Input: part model. Units: mm. Frame: model coordinates. A direction names the side the tool comes from. Round coordinates to 2 decimals unless told otherwise and drop trailing zeros. Loops run counter-clockwise (first coordinate to the right, second up) from the corner with the lowest first, then second, coordinate; pieces in that order, holes last. Notation, with made-up numbers: (34, 39) -> (49, 39) arc R16 cw to (49, 63) -> close; hole circle Ø11 at (16.5, 70.5). An arc over 180 degrees is marked (long way). Answer as a JSON object with one key per item and string values. Group by question number.
Item 1: Section query C-C on z = 15.25. Count the separate pieces of the cut face and the enclosed holes in it, and give its area (3 significant figures).
Item 2: Material intervals for line 1 (Y direction, x = 44, z = 6.75); line 2 (X direction, y = 22, z = 8.5); line 3 (X direction, y = 12, z = 15), sorted ascending. Write a range as [from, to].
Item 3: Section query B-B on y = 7.5. Return loops of the section in (x, z), and give its area (3 significant figures).
Item 4: Pin query (flat end, axial travel): pin 1 (19 mm diameter, centred on x = 2, y = 84, fed in from -Z); pin 2 (1.5 mm diameter, centred on x = 32, y = 17.5, fed in from -Z); pin 3 (1 mm diameter, centred on y = -23.5, z = 7, fed in from -X); pin 4 (2 mm diameter, centred on x = -16, z = 21.5, fed in from +Y). Return the tip coordinate at first contact, or that it passes through.
Item 5: Section query A-A on x = 18. Return loops of the section in (y, z), and give its area (3 significant figures).
Item 6: Set-up query: faces 3 (the cylindrical face through (-0.16, 87.21, 22.48)), 4 (the flat face through (-2, 85, 12)), 5 (the cylindrical face through (-0.19, 87.21, 3.04)), 6 (the flat face through (-1, -31.105, 12)). Return all of +Z, -Z, +X, -X, +Y, -Y with unobstructed straight access to the full face (end or side cutting, diameter ignored); none if empty.
Item 7: Draft query along Y for faces 1 (the flat face through (-20.54, 66.63, 18.6)), 2 (the flat face through (-30, 13, 0)). Return one class per face: released by +Y, released by -Y, zero draft, split by the parting line, or undercut.
from build123d import *

# Parameters (mm, degrees)
PAD_DEPTH             = 24
POCKET_DEPTH          = 3
SKETCH002_W           = 70
SKETCH002_H           = 18.5
POCKET001_DEPTH       = 18
POLARPATTERN_COUNT    = 3
POCKET002_DEPTH       = 6
CHAMFER_SIZE          = 8
FILLET_R              = 13
FILLET001_R           = 11
CHAMFER001_SIZE       = 16.1
FILLET002_R           = 11
FILLET003_R           = 12
POCKET003_DEPTH       = 6
POCKET004_DEPTH       = 18
POCKET005_DEPTH       = 21.001
SKETCH007_W           = 15.5
SKETCH007_H           = 15
POCKET006_DEPTH       = 5
SKETCH010_W           = 13.6
SKETCH010_H           = 9
POCKET009_DEPTH       = 15.5
POCKET010_DEPTH       = 3
SKETCH012_R           = 1.85
SKETCH012_R_2         = 0.99
POCKET011_DEPTH       = 498.0492855781
POLARPATTERN001_COUNT = 3


with BuildPart() as part:
    # Sketch → Pad (new body)
    with BuildSketch(Plane.XY):
        Polygon((0, 112.2094915052), (-97.1762701892, -56.1047457526), (97.1762701892, -56.1047457526), align=None)
        Polygon((0, 62.2094915052), (-53.875, -31.1047457526), (53.875, -31.1047457526), align=None, mode=Mode.SUBTRACT)
    extrude(amount=PAD_DEPTH)

    # Sketch001 (on Face8 of Pad) → Pocket (cut)
    with BuildSketch(Plane.XY.offset(24)):
        Polygon((0, 98.2094915052), (-85.0519145362, -49.1047457526), (85.0519145362, -49.1047457526), align=None)
        Polygon((0, 76.2094915052), (-65.999355653, -38.1047457526), (65.999355653, -38.1047457526), align=None, mode=Mode.SUBTRACT)
    extrude(amount=-POCKET_DEPTH, mode=Mode.SUBTRACT)

    # Sketch002 (on Face4 of Pocket) → Pocket001 (cut)
    with BuildSketch(Plane(origin=(0, 0, 0), x_dir=(1, 0, 0), z_dir=(0, 0, -1))):
        with Locations((0, 43.6047457526)):
            Rectangle(SKETCH002_W, SKETCH002_H)
    pocket001 = extrude(amount=-POCKET001_DEPTH, mode=Mode.SUBTRACT)

    # PolarPattern: Pocket001 ×3 about axis
    polarpattern_axis = Axis((0, 0, 0), (0, 0, -1))
    for i in range(1, POLARPATTERN_COUNT):
        add(pocket001.rotate(polarpattern_axis, i * 360 / POLARPATTERN_COUNT), mode=Mode.SUBTRACT)

    # Sketch003 (on Face4 of PolarPattern) → Pocket002 (cut)
    with BuildSketch(Plane(origin=(0, 0, 0), x_dir=(1, 0, 0), z_dir=(0, 0, -1))):
        Polygon((0, -100.2094915052), (86.7839653438, 50.1047457526), (-86.7839653438, 50.1047457526), align=None)
        Polygon((0, -74.2094915052), (64.2673048454, 37.1047457526), (-64.2673048454, 37.1047457526), align=None, mode=Mode.SUBTRACT)
    extrude(amount=-POCKET002_DEPTH, mode=Mode.SUBTRACT)

    # Chamfer
    chamfer_edges = [part.edges().sort_by_distance(p)[0] for p in [
        (-53.875, -31.104746, 12),
        (53.875, -31.104746, 12),
        (0, 62.209492, 12),
    ]]
    chamfer(chamfer_edges, length=CHAMFER_SIZE)

    # Fillet
    fillet_edges = [part.edges().sort_by_distance(p)[0] for p in [
        (0, 100.209492, 3),
        (-86.783965, -50.104746, 3),
        (86.783965, -50.104746, 3),
    ]]
    fillet(fillet_edges, radius=FILLET_R)

    # Fillet001
    fillet001_edges = [part.edges().sort_by_distance(p)[0] for p in [
        (0, 74.209492, 3),
        (64.267305, -37.104746, 3),
        (-64.267305, -37.104746, 3),
    ]]
    fillet(fillet001_edges, radius=FILLET001_R)

    # Chamfer001
    chamfer001_edges = [part.edges().sort_by_distance(p)[0] for p in [
        (97.17627, -56.104746, 12),
        (0, 112.209492, 12),
        (-97.17627, -56.104746, 12),
    ]]
    chamfer(chamfer001_edges, length=CHAMFER001_SIZE)

    # Fillet002
    fillet002_edges = [part.edges().sort_by_distance(p)[0] for p in [
        (0, 98.209492, 22.5),
        (-85.051915, -49.104746, 22.5),
        (85.051915, -49.104746, 22.5),
    ]]
    fillet(fillet002_edges, radius=FILLET002_R)

    # Fillet003
    fillet003_edges = [part.edges().sort_by_distance(p)[0] for p in [
        (65.999356, -38.104746, 22.5),
        (0, 76.209492, 22.5),
        (-65.999356, -38.104746, 22.5),
    ]]
    fillet(fillet003_edges, radius=FILLET003_R)

    # Sketch004 (on Face60 of Fillet003) → Pocket003 (cut)
    with BuildSketch(Plane(origin=(0, 0, 6), x_dir=(1, 0, 0), z_dir=(0, 0, -1))):
        Polygon((-8.75, -71.2664825043), (8.75, -71.2664825043), (8.75, -94.7664825043), (4, -94.7664825043), (4, -98.2664825043), (-4, -98.2664825043), (-4, -94.7664825043), (-8.75, -94.7664825043), align=None)
    extrude(amount=-POCKET003_DEPTH, mode=Mode.SUBTRACT)

    # Sketch005 (on Face29 of Pocket003) → Pocket004 (cut)
    with BuildSketch(Plane(origin=(0, 0, 0), x_dir=(1, 0, 0), z_dir=(0, 0, -1))):
        Polygon((46.1715988394, 38.9547457526), (68.6882593378, 51.9547457526), (79.3382593378, 33.508404652), (56.8215988394, 20.508404652), align=None)
    extrude(amount=-POCKET004_DEPTH, mode=Mode.SUBTRACT)

    # Sketch006 (on Face1 of Pocket004) → Pocket005 (cut, through all)
    with BuildSketch(Plane.XY.offset(21)):
        with BuildLine():
            ThreePointArc((1.5, 85.0404521425), (0, 86.5404521425), (-1.5, 85.0404521425))
            Line((-1.5, 85.0404521425), (-1.5, 66.0404521425))
            ThreePointArc((-1.5, 66.0404521425), (0, 64.5404521425), (1.5, 66.0404521425))
            Line((1.5, 85.0404521425), (1.5, 66.0404521425))
        make_face()
    extrude(amount=-POCKET005_DEPTH, mode=Mode.SUBTRACT)

    # Sketch007 (on Face24 of Pocket005) → Pocket006 (cut)
    with BuildSketch(Plane(origin=(-48.5881350946, 28.0523728763, 0), x_dir=(-0.5, -0.8660254038, 0), z_dir=(-0.8660254038, 0.5, 0))):
        with Locations((-47.3262701892, 13.5)):
            Rectangle(SKETCH007_W, SKETCH007_H)
    extrude(amount=-POCKET006_DEPTH, mode=Mode.SUBTRACT)

    # Sketch010 (on Face79 of Pocket006) → Pocket009 (cut)
    with BuildSketch(Plane(origin=(-44.2580080757, 25.5523728763, 0), x_dir=(-0.5, -0.8660254038, 0), z_dir=(-0.8660254038, 0.5, 0))):
        with Locations((-47.3262701892, 13.5)):
            Rectangle(SKETCH010_W, SKETCH010_H)
    extrude(amount=-POCKET009_DEPTH, mode=Mode.SUBTRACT)

    # Sketch011 (on Face21 of Pocket009) → Pocket010 (cut)
    with BuildSketch(Plane(origin=(0, 0, 6), x_dir=(1, 0, 0), z_dir=(0, 0, -1))):
        Polygon((-21.0413798427, -59.7570681827), (-11.6817654684, -54.3532923042), (-6.658482036, -63.0538744299), (-16.0180964103, -68.4576503084), align=None)
    extrude(amount=-POCKET010_DEPTH, mode=Mode.SUBTRACT)

    # Sketch012 (on Face54 of Pocket010) → Pocket011 (cut, through all)
    with BuildSketch(Plane(origin=(0, 0, 0), x_dir=(1, 0, 0), z_dir=(0, 0, -1))):
        with Locations((-13.5, -82.7032108255)):
            Circle(SKETCH012_R)
        with Locations((13.5, -82.7032108255)):
            Circle(SKETCH012_R)
        with Locations((-6.25, -96.5164825043)):
            Circle(SKETCH012_R_2)
        with Locations((6.25, -96.5164825043)):
            Circle(SKETCH012_R_2)
        with Locations((-27.2463245869, -59.0174730012)):
            Circle(SKETCH012_R_2)
        with Locations((-47.1862074814, -27.2405827309)):
            Circle(SKETCH012_R_2)
        with Locations((-64.7337931796, 5.9127272486)):
            Circle(SKETCH012_R_2)
        with Locations((-10.791841915, -49.5174730012)):
            Circle(SKETCH012_R_2)
        with Locations((-28.3394276132, -16.3641630217)):
            Circle(SKETCH012_R_2)
        with Locations((-48.2793105078, 15.4127272487)):
            Circle(SKETCH012_R_2)
    pocket011 = extrude(amount=-POCKET011_DEPTH, mode=Mode.SUBTRACT)

    # PolarPattern001: Pocket011 ×3 about axis
    polarpattern001_axis = Axis((0, 0, 0), (0, 0, -1))
    for i in range(1, POLARPATTERN001_COUNT):
        add(pocket011.rotate(polarpattern001_axis, i * 360 / POLARPATTERN001_COUNT), mode=Mode.SUBTRACT)


solid = part.part
Solved:
{
 "1": {"separate pieces": "1", "enclosed holes": "36", "area": "6,150 mm²"},
 "2": {"line 1": "[-56.1, -31.1], [-14, -7.5], [29.5, 36]", "line 2": "[-52.08, -48.33], [-26.97, -23.21], [23.21, 26.97], [48.33, 52.08]", "line 3": "[-57.86, -54.1], [-32.74, -28.99], [28.99, 32.74], [54.1, 57.86]"},
 "3": {"outline": "(-60.45, 0) -> (-56.7, 0) -> (-56.7, 18) -> (-35.34, 18) -> (-35.34, 0) -> (-31.59, 0) -> (-31.59, 24) -> (-39.67, 24) -> (-39.67, 21) -> (-52.37, 21) -> (-52.37, 24) -> (-60.45, 24) -> close; (31.59, 0) -> (35.34, 0) -> (35.34, 18) -> (56.7, 18) -> (56.7, 0) -> (60.45, 0) -> (60.45, 24) -> (52.37, 24) -> (52.37, 21) -> (39.67, 21) -> (39.67, 24) -> (31.59, 24) -> close", "area": "540 mm²"},
 "4": {"pin 1": "z = 0", "pin 2": "z = 18", "pin 3": "x = -78.64", "pin 4": "y = 86.23"},
 "5": {"outline": "(-56.1, 0) -> (-52.85, 0) -> (-52.85, 18) -> (-34.35, 18) -> (-34.35, 0) -> (-31.1, 0) -> (-31.1, 24) -> (-38.1, 24) -> (-38.1, 21) -> (-49.1, 21) -> (-49.1, 24) -> (-56.1, 24) -> close; (31.03, 0) -> (37.53, 0) -> (37.53, 18) -> (50.81, 18) -> (50.81, 6) -> (69.03, 6) -> (69.03, 0) -> (81.03, 0) -> (81.03, 24) -> (67.03, 24) -> (67.03, 21) -> (45.03, 21) -> (45.03, 24) -> (31.03, 24) -> close", "area": "1,020 mm²"},
 "6": {"face 3": "+Z", "face 4": "none", "face 5": "-Z", "face 6": "+Z, -Z"},
 "7": {"face 1": "undercut", "face 2": "zero draft"}
}
